Answer from the drawing. Dimensions are ordinates in mm from the lowest x, y and z of the part. A direction names the side the tool comes from. Coordinates: 2 decimals unless noted, no trailing zeros. Loops run counter-clockwise (first coordinate to the right, second up) from the corner with the lowest first, then second, coordinate; pieces in that order, holes last. Notation, with made-up numbers: (-9.75, 41.25) -> (-5.75, 41.25) arc R9 ccw to (-5.75, 51.25) -> close; hole circle Ø3 at (41.5, 60.25). An arc over 180 degrees is marked (long way). Use a Markdown table: item, result.
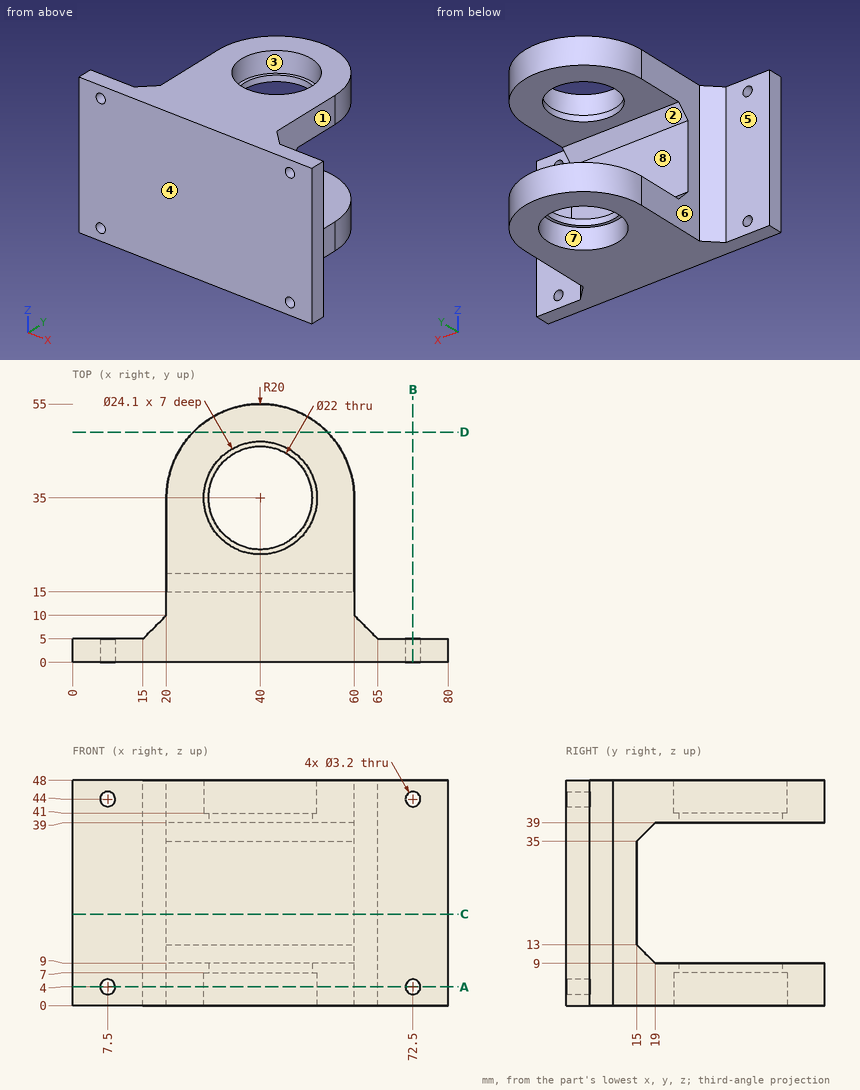
Q1. Section A-A on z = 4 is taken. Determine the outline of the cut face in (x, y).
Solved:
| item | result |
|---|---|
| outline | (0, 0) -> (5.9, 0) -> (5.9, 5) -> (0, 5) -> close; (9.1, 0) -> (70.9, 0) -> (70.9, 5) -> (65, 5) -> (60, 10) -> (60, 35) arc R20 ccw to (20, 35) -> (20, 10) -> (15, 5) -> (9.1, 5) -> close; (74.1, 0) -> (80, 0) -> (80, 5) -> (74.1, 5) -> close; hole circle Ø24.1 at (40, 35) |
Q2. Section C-C on z = 19.5 is taken. Determine the outline of the cut face in (x, y), and give its area (3 significant figures).
Solved:
| item | result |
|---|---|
| outline | (0, 0) -> (80, 0) -> (80, 5) -> (65, 5) -> (60, 10) -> (60, 15) -> (20, 15) -> (20, 10) -> (15, 5) -> (0, 5) -> close |
| area | 825 mm² |
Q3. Section B-B on x = 72.5 is taken. Determine the outline of the cut face in (y, z).
Solved:
| item | result |
|---|---|
| outline | (0, 0) -> (5, 0) -> (5, 2.4) -> (0, 2.4) -> close; (0, 5.6) -> (5, 5.6) -> (5, 42.4) -> (0, 42.4) -> close; (0, 45.6) -> (5, 45.6) -> (5, 48) -> (0, 48) -> close |
Q4. For the marked faces 1, 2, 3, 4 and 5, determine the directions among +Z, -Z, +X, -X, +Y, -Y from which every point of the face is accessible in a straight line to the end or side of a thin tool.
Solved:
| item | result |
|---|---|
| face 1 | +Z, -Z, +X, +Y |
| face 2 | +X, -X, +Y |
| face 3 | +Z |
| face 4 | +Z, -Z, +X, -X, -Y |
| face 5 | +Z, -Z, -X, +Y |
Q5. Determine the mould class of the marked faces 6, 7 and 8 for opening direction X: pulls with the +X half, pulls with the -X half, needs draft (parallel to the pull), parting line crosses it, or undercut.
Solved:
| item | result |
|---|---|
| face 6 | pulls with the -X half |
| face 7 | undercut |
| face 8 | needs draft |
Q6. Section D-D on y = 49 is taken. Determine the outline of the cut face in (x, z), and give its area (3 significant figures).
Solved:
| item | result |
|---|---|
| outline | (25.72, 0) -> (54.28, 0) -> (54.28, 9) -> (25.72, 9) -> close; (25.72, 39) -> (54.28, 39) -> (54.28, 48) -> (25.72, 48) -> close |
| area | 514 mm² |
Q7. Consider line 1 (X direction, y = 35, z = 8); line 2 (X direction, y = 2.65, z = 4); line 3 (Y direction, x = 71, z = 26.5). Determine where each line is inside the solid, lowest interval first. Write a range as [from, to].
Solved:
| item | result |
|---|---|
| line 1 | [20, 29], [51, 60] |
| line 2 | [0, 5.9], [9.1, 70.9], [74.1, 80] |
| line 3 | [0, 5] |
Q8. Given pin 1 Ø10 at (x, z) = (18.5, 41) entering from +Y; pin 2 Ø1.9 at (x, z) = (7.5, 44) entering from +Y; pin 3 Ø24 at (x, z) = (35, 23) entering from +Y; pin 4 Ø7.5 at (x, z) = (5, 27.5) entering from +Y, each flat-ended and moving along its own axis, determine where each tip first touches the part or whether it passes through.
Solved:
| item | result |
|---|---|
| pin 1 | y = 46.3 |
| pin 2 | through |
| pin 3 | y = 17 |
| pin 4 | y = 5 |
